Design review of the part built by this model. Coordinates are the model's own, in mm. Face numbers are marked on the shaded views. A direction names the side the tool comes from. Coordinates: 2 decimals unless noted, no trailing zeros. Loops run counter-clockwise (first coordinate to the right, second up) from the corner with the lowest first, then second, coordinate; pieces in that order, holes last. Notation, with made-up numbers: (89.25, 76) -> (93.25, 76) arc R26 cw to (93.25, 93) -> close; hole circle Ø4 at (-6.75, 77.5). An arc over 180 degrees is marked (long way). Use a Markdown table: item, result. Add a question column.
Q1. Take a section at D-D on x = 5. Write out the cut boundary in (y, z), plus the area to 3 significant figures.
Q2. For the marked faces 4 and 5, list the 3-axis set-ups (+Z, -Z, +X, -X, +Y, -Y) from which the entire face can be reached by the end or side of a thin tool; tool diameter is ignored.
Q3. Clearance check with flat-ended pins moving along their axes: pin 1 Ø1.1 at (x, y) = (6.75, 16) entering from -Z; pin 2 Ø0.6 at (x, z) = (5, 1) entering from -Y. State where each tip first meets the part, or that it passes through.
Q4. Take a section at B-B on y = 10. Write out the cut boundary in (x, z), plus the area to 3 significant figures.
Q5. For probe 1 along Y at (x, z) = (9.75, 1.9); probe 2 along Y at (x, z) = (17.25, 0.75); probe 3 along X at (y, z) = (13.5, 1.3), list the stretches that pass through material, from the lowest coordinate up.
Q6. Take a section at C-C on z = 0.3. Write out the cut boundary in (x, y).
Q7. Draft analysis for pull direction X (two halves, no side actions). For the marked faces 1, 2 and 3, state which applies: pulls with the +X half, pulls with the -X half, needs draft (parallel to the pull), parting line crosses it, or undercut.
Q8. Take a section at A-A on x = 17.25. Write out the cut boundary in (y, z).
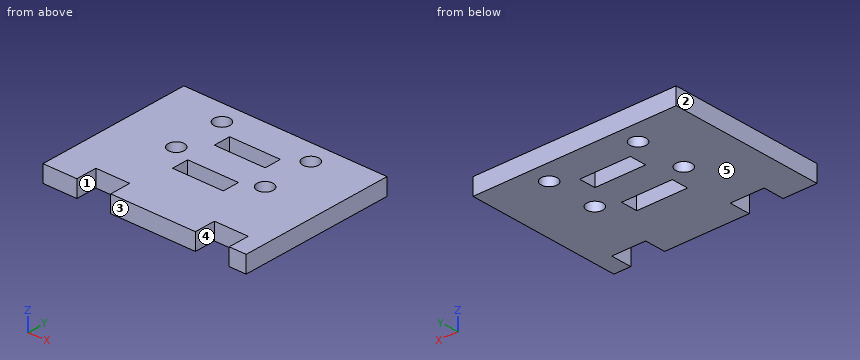
from build123d import *

# Parameters (mm, degrees)
SKETCH1_R           = 0.95
SKETCH1_W           = 6
SKETCH1_H           = 2
BOSS_EXTRUDE1_DEPTH = 2


with BuildPart() as part:
    # Sketch1 → Boss-Extrude1 (new body)
    with BuildSketch(Plane.XY):
        Polygon((4, 2.5), (8, 2.5), (8, 0), (18, 0), (18, 2.5), (22, 2.5), (22, 0), (24, 0), (24, 18.5), (0, 18.5), (0, 0), (4, 0), align=None)
        with Locations((6.75, 16)):
            Circle(SKETCH1_R, mode=Mode.SUBTRACT)
        with Locations((17.25, 10)):
            Circle(SKETCH1_R, mode=Mode.SUBTRACT)
        with Locations((17.25, 16)):
            Circle(SKETCH1_R, mode=Mode.SUBTRACT)
        with Locations((6.75, 10)):
            Circle(SKETCH1_R, mode=Mode.SUBTRACT)
        with Locations((12, 13.5)):
            Rectangle(SKETCH1_W, SKETCH1_H, mode=Mode.SUBTRACT)
        with Locations((12, 8)):
            Rectangle(SKETCH1_W, SKETCH1_H, mode=Mode.SUBTRACT)
    extrude(amount=BOSS_EXTRUDE1_DEPTH)


solid = part.part
Answer list:
| question | item | result |
|---|---|---|
| 1 | outline | (2.5, 0) -> (18.5, 0) -> (18.5, 2) -> (2.5, 2) -> close |
| 1 | area | 32.0 mm² |
| 2 | face 4 | +Z, -Z, -Y |
| 2 | face 5 | -Z, +X, -X, +Y, -Y |
| 3 | pin 1 | through |
| 3 | pin 2 | y = 2.5 |
| 4 | outline | (0, 0) -> (5.8, 0) -> (5.8, 2) -> (0, 2) -> close; (7.7, 0) -> (16.3, 0) -> (16.3, 2) -> (7.7, 2) -> close; (18.2, 0) -> (24, 0) -> (24, 2) -> (18.2, 2) -> close |
| 4 | area | 40.4 mm² |
| 5 | probe 1 | 0 to 7, 9 to 12.5, 14.5 to 18.5 |
| 5 | probe 2 | 0 to 9.05, 10.95 to 15.05, 16.95 to 18.5 |
| 5 | probe 3 | 0 to 9, 15 to 24 |
| 6 | outline | (0, 0) -> (4, 0) -> (4, 2.5) -> (8, 2.5) -> (8, 0) -> (18, 0) -> (18, 2.5) -> (22, 2.5) -> (22, 0) -> (24, 0) -> (24, 18.5) -> (0, 18.5) -> close; hole circle Ø1.9 at (6.75, 10); hole circle Ø1.9 at (6.75, 16); hole (9, 7) -> (15, 7) -> (15, 9) -> (9, 9) -> close; hole (9, 12.5) -> (15, 12.5) -> (15, 14.5) -> (9, 14.5) -> close; hole circle Ø1.9 at (17.25, 10); hole circle Ø1.9 at (17.25, 16) |
| 7 | face 1 | undercut |
| 7 | face 2 | pulls with the -X half |
| 7 | face 3 | needs draft |
| 8 | outline | (0, 0) -> (9.05, 0) -> (9.05, 2) -> (0, 2) -> close; (10.95, 0) -> (15.05, 0) -> (15.05, 2) -> (10.95, 2) -> close; (16.95, 0) -> (18.5, 0) -> (18.5, 2) -> (16.95, 2) -> close |
